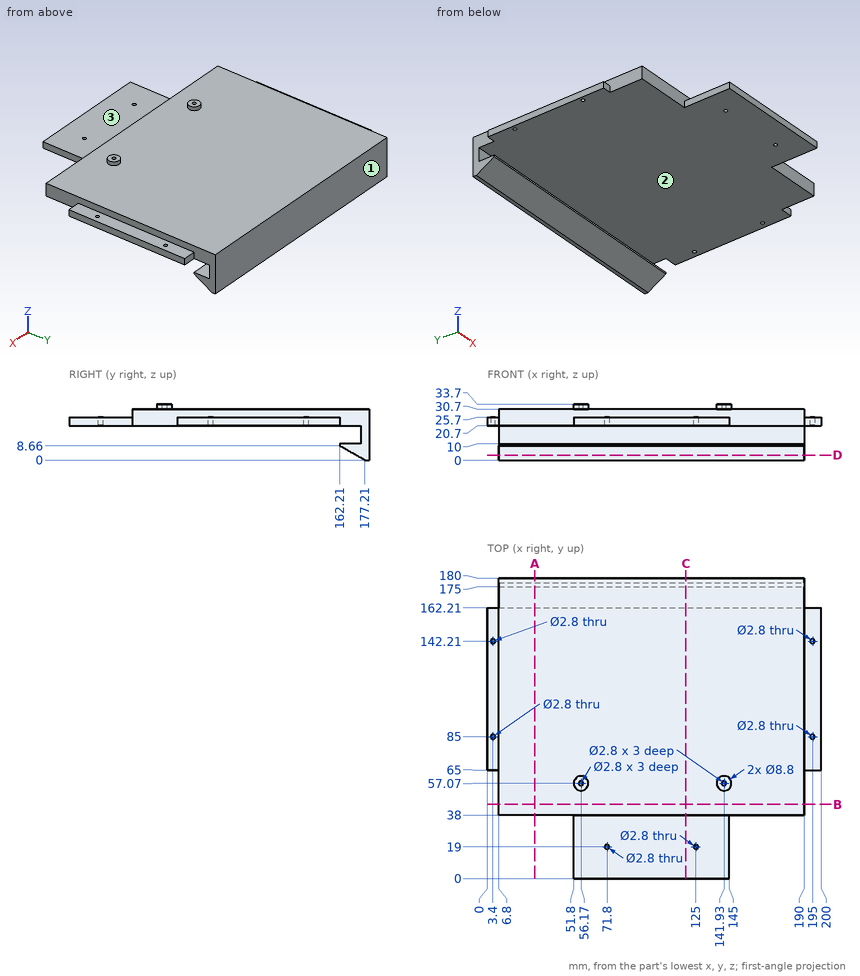
The figure shows three views and two pictorial views of one solid part (mm, origin at its lowest corner). Answer the questions. A direction names the side the tool comes from. Coordinates: 2 decimals unless noted, no trailing zeros. Loops run counter-clockwise (first coordinate to the right, second up) from the corner with the lowest first, then second, coordinate; pieces in that order, holes last.
(1) The part is cut by section C-C (x = 119). Determine the outline of the cut face in (y, z), and give its area (3 significant figures).
Solution:
outline: (0, 20.7) - (175, 20.7) - (175, 10) - (162.21, 10) - (162.21, 8.66) - (177.21, 0) - (180, 0) - (180, 30.7) - (38, 30.7) - (38, 25.7) - (0, 25.7) - close
area: 1,780 mm2
(2) Consider line 1 along Y through (x, z) = (3.4, 23.6); line 2 along X through (y, z) = (85, 24.35); line 3 along Z through (x, y) = (117, 99.5). Determine where each line is inside the solid, lowest interval first.
Solution:
line 1: y = 65 to 83.6, 86.4 to 140.81, 143.61 to 162.21
line 2: x = 0 to 2, 4.8 to 193.6, 196.4 to 200
line 3: z = 20.7 to 30.7
(3) The part is cut by section B-B (y = 44.5). Determine the outline of the cut face in (x, z), and give its area (3 significant figures).
Solution:
outline: (6.8, 20.7) - (190, 20.7) - (190, 30.7) - (6.8, 30.7) - close
area: 1,830 mm2
(4) Flat-ended cylindrical pins translate along their axes: pin 1 Ø4 at (x, y) = (140, 101.5) entering from -Z; pin 2 Ø11.5 at (x, y) = (117.5, 26) entering from +Z; pin 3 Ø4 at (x, z) = (193, 23.5) entering from -Y. Find the tip coordinate at first contact, or state that the pin passes through.
Solution:
pin 1: stops at z = 20.7
pin 2: stops at z = 25.7
pin 3: stops at y = 65
(5) A tool of negligible diameter and unlimited length cuts with its end or side. For the marked faces 1, 2 and 3, from which of +Z, -Z, +X, -X, +Y, -Y can it reach the whole face along a straight path? Write none if from no direction.
Solution:
face 1: +Z, -Z, +X, -X, +Y
face 2: +X, -X, -Y
face 3: +Z, +X, -X, -Y
(6) The part is cut by section A-A (x = 28.5). Determine the outline of the cut face in (y, z).
Solution:
outline: (38, 20.7) - (175, 20.7) - (175, 10) - (162.21, 10) - (162.21, 8.66) - (177.21, 0) - (180, 0) - (180, 30.7) - (38, 30.7) - close
(7) The part is cut by section D-D (z = 3). Determine the outline of the cut face in (x, y), and give its area (3 significant figures).
Solution:
outline: (6.8, 172.01) - (190, 172.01) - (190, 180) - (6.8, 180) - close
area: 1,460 mm2
